```python
from build123d import *


with BuildPart() as part:
    # Sketch 1 → Revolve 1 (revolve)
    with BuildSketch(Plane.XY, mode=Mode.PRIVATE) as revolve_1_sk:
        with BuildLine():
            Line((0, 0), (0, 7.85))
            Line((0, 7.85), (4.1, 7.85))
            Line((4.1, 7.85), (11.8, 4.85))
            Line((11.8, 4.85), (13.20030223, 4.85))
            ThreePointArc((13.20030223, 4.85), (16.597019137, 6.257515188), (20.2, 5.524498371))
            Line((20.2, 5.524498371), (20.2, 0))
            Line((20.2, 0), (0, 0))
        make_face()
    revolve(revolve_1_sk.sketch.rotate(Axis((20.2, 0, 0), (-1, 0, 0)), 270), axis=Axis((20.2, 0, 0), (-1, 0, 0)))

    # Sketch 2 → Cut-Revolve 1 (revolve, cut)
    with BuildSketch(Plane.XY):
        with BuildLine():
            Line((8.9865, 0), (-3.5865, 0))
            ThreePointArc((-3.5865, 0), (2.7, 6.2865), (8.9865, 0))
        make_face()
    revolve(axis=Axis((50, 0, 0), (-1, 0, 0)), mode=Mode.SUBTRACT)


solid = part.part
```
Here's how the part is built. I have some questions about the finished solid (model axes, mm). Round coordinates to 2 decimals unless told otherwise and drop trailing zeros. Order: outer loops, then holes, each group sorted by start corner. A loop starts at its lowest first (then second) coordinate and runs counter-clockwise, first axis right, second up. Notation, with made-up numbers: M 28,11 L 72,11 A17 ccw 72,33 Z; hole C 35,87.5 d1. An arc over 180 degrees is marked long. Answer as CSV lines item,"result".
Item 1: Imagine slicing it at A-A on z = 0. List the corners of the cut face in (x, y) for me.
From the geometry:
outline,"M 0,-7.85 L 4.1,-7.85 L 11.8,-4.85 L 13.2,-4.85 A6.29 ccw 20.2,-5.52 L 20.2,5.52 A6.29 ccw 13.2,4.85 L 11.8,4.85 L 4.1,7.85 L 0,7.85 L 0,5.68 A6.29 cw long 0,-5.68 Z"
Item 2: Imagine slicing it at D-D on x = 10.5. List the corners of the cut face in (y, z) for me, and give its area (3 significant figures).
From the geometry:
outline,"C 0,0 d10.71"
area,"90.1 mm2"
Item 3: We'd pull the mould along X, two halves only. Please class faces 1 (the conical face through (10.571, -2.041, 4.923)), 2 (the cylindrical face through (12.51, 1.457, 4.626)), 3 (the cylindrical face through (2.079, -4.777, -6.229)), 4 (the flat face through (20.2, 0, 0)): +X half, -X half, draft (parallel to the pull), parting line (faces both ways), or undercut.
From the geometry:
face 1,"undercut"
face 2,"undercut"
face 3,"draft"
face 4,"+X half"
Item 4: For pin 1 (1 mm diameter, centred on x = 4.5, y = -0.5, fed in from -Z); pin 2 (2 mm diameter, centred on x = 3, y = -3.5, fed in from +Z), each with a flat end and sliding along its axis, tell me the tip position at first contact or that it passes through.
From the geometry:
pin 1,"z = -7.85"
pin 2,"z = 7.44"
Item 5: Please list where these lines run through material, in increasing order: L1, parallel to Y at x = 6.75, z = -1; L2, parallel to Z at x = 14.25, y = 0.5; L3, parallel to Y at x = 11.5, z = -1.5. Write a range as [from, to].
From the geometry:
L1,"[-6.74, -4.7], [4.7, 6.74]"
L2,"[-5.53, 5.53]"
L3,"[-4.73, 4.73]"
Item 6: Imagine slicing it at B-B on z = 6. Give the number of separate pieces and of enclosed holes in the cut face, and give its area (3 significant figures).
From the geometry:
separate pieces,"2"
enclosed holes,"1"
area,"72.7 mm2"
